```python
from build123d import *

# Parameters (mm, degrees)
SKETCH1_R           = 3.75
BOSS_EXTRUDE1_DEPTH = 7.25
SKETCH3_R           = 3.75
SKETCH3_R_2         = 3.25
CUT_EXTRUDE1_DEPTH  = 2
SKETCH4_R           = 1.75
CUT_EXTRUDE2_DEPTH  = 6.75
SKETCH5_R           = 2.5
CUT_EXTRUDE3_DEPTH  = 1


with BuildPart() as part:
    # Sketch1 → Boss-Extrude1 (new body)
    with BuildSketch(Plane(origin=(0, 0, 0), x_dir=(1, 0, 0), z_dir=(0, 1, 0))):
        Circle(SKETCH1_R)
    extrude(amount=BOSS_EXTRUDE1_DEPTH)

    # Sketch3 → Cut-Extrude1 (cut)
    with BuildSketch(Plane(origin=(0, 7.25, 0), x_dir=(1, 0, 0), z_dir=(0, 1, 0))):
        Circle(SKETCH3_R)
        Circle(SKETCH3_R_2, mode=Mode.SUBTRACT)
    extrude(amount=-CUT_EXTRUDE1_DEPTH, mode=Mode.SUBTRACT)

    # Sketch4 → Cut-Extrude2 (cut)
    with BuildSketch(Plane(origin=(0, 7.25, 0), x_dir=(1, 0, 0), z_dir=(0, 1, 0))):
        Circle(SKETCH4_R)
    extrude(amount=-CUT_EXTRUDE2_DEPTH, mode=Mode.SUBTRACT)

    # Sketch5 → Cut-Extrude3 (cut)
    with BuildSketch(Plane(origin=(0, 7.25, 0), x_dir=(1, 0, 0), z_dir=(0, 1, 0))):
        Circle(SKETCH5_R)
    extrude(amount=-CUT_EXTRUDE3_DEPTH, mode=Mode.SUBTRACT)


solid = part.part
```
Check sheet for the modelled part. Datum: model origin and axes. Units: mm. A direction names the side the tool comes from. Round coordinates to 2 decimals unless told otherwise and drop trailing zeros. Order: outer loops, then holes, each group sorted by start corner. A loop starts at its lowest first (then second) coordinate and runs counter-clockwise, first axis right, second up. Notation, with made-up numbers: (24.5, 50.25) - (35.5, 50.25) arc R16 cw to (35.5, 75.25) - close; hole circle Ø10 at (-35, -40). An arc over 180 degrees is marked (long way). Write item = value, one per line.
Q1. Thickness scan on line 1 along Z through (x, y) = (0, 3.95); line 2 along Z through (x, y) = (0, 6.85). Record the ranges inside material, lowest first.
Computed:
line_1 = -3.75 to -1.75, 1.75 to 3.75
line_2 = -3.25 to -2.5, 2.5 to 3.25
Q2. Tool access check on faces 5 (the face through (1.617, 3.415, 0.67)), 6 (the face through (-3.746, 2.588, -0.165)). Record the directions out of +Z, -Z, +X, -X, +Y, -Y that give a thin tool (end or side, any length) a straight path to the whole face; none if there is none.
Computed:
face_5 = +Y
face_6 = +Y, -Y
Q3. Draft check along X on faces 1 (the face through (-2, 6.25, 1)), 2 (the face through (0, 0, 0)), 3 (the face through (-0.54, 6.76, 2.44)), 4 (the face through (-2.579, 6.264, 1.978)). Enter one of: pulls with the +X half, pulls with the -X half, needs draft (parallel to the pull), parting line crosses it, or undercut.
Computed:
face_1 = undercut
face_2 = needs draft
face_3 = undercut
face_4 = parting line crosses it
Q4. Section check B-B (z = 0). Record the boundary of the cut face in (x, y), and give its area (4 significant figures).
Computed:
outline = (-3.75, 0) - (3.75, 0) - (3.75, 5.25) - (3.25, 5.25) - (3.25, 7.25) - (2.5, 7.25) - (2.5, 6.25) - (1.75, 6.25) - (1.75, 0.5) - (-1.75, 0.5) - (-1.75, 6.25) - (-2.5, 6.25) - (-2.5, 7.25) - (-3.25, 7.25) - (-3.25, 5.25) - (-3.75, 5.25) - close
area = 27.25 mm^2
Q5. Section check A-A (x = 0). Record the boundary of the cut face in (y, z).
Computed:
outline = (0, -3.75) - (5.25, -3.75) - (5.25, -3.25) - (7.25, -3.25) - (7.25, -2.5) - (6.25, -2.5) - (6.25, -1.75) - (0.5, -1.75) - (0.5, 1.75) - (6.25, 1.75) - (6.25, 2.5) - (7.25, 2.5) - (7.25, 3.25) - (5.25, 3.25) - (5.25, 3.75) - (0, 3.75) - close
Q6. Section check C-C (y = 5). Record the boundary of the cut face in (x, z), and give its area (3 significant figures).
Computed:
outline = circle Ø7.5 at (0, 0); hole circle Ø3.5 at (0, 0)
area = 34.6 mm^2
Q7. Section check D-D (y = 6). Record the boundary of the cut face in (x, z).
Computed:
outline = circle Ø6.5 at (0, 0); hole circle Ø3.5 at (0, 0)
Q8. Go/stop test with flat-tipped pins: pin 1 (1 mm diameter, centred on x = -2.5, y = 6, fed in from -Z); pin 2 (3 mm diameter, centred on x = 2.5, y = 6, fed in from -Z); pin 3 (3 mm diameter, centred on x = -0.5, z = -0.5, fed in from +Y). Record where each tip stops, or that it passes through.
Computed:
pin_1 = -2.56
pin_2 = -3.55
pin_3 = 6.25
